Check sheet for the modelled part. Datum: model origin and axes. Units: mm. Face numbers are marked on the shaded views. A direction names the side the tool comes from. Give positions to 0.01 mm unless a question says otherwise; leave off trailing zeros. Order: outer loops, then holes, each group sorted by start corner. A loop starts at its lowest first (then second) coordinate and runs counter-clockwise, first axis right, second up.
from build123d import *

# Parameters (mm, degrees)
F0_R     = 11
F1_DEPTH = 7


with BuildPart() as f1:
    # F0 (on Top) → F1 (new body)
    with BuildSketch(Plane.XY):
        with BuildLine():
            ThreePointArc((-2.577571, 23.56544), (0.124952, 23.151761), (2.813649, 23.647409))
            ThreePointArc((2.813649, 23.647409), (6.73351, 26.656757), (8.219155, 31.369967))
            ThreePointArc((8.219155, 31.369967), (-4.815031, 38.031046), (-2.577571, 23.56544))
        make_face()
        Polygon((6.520027, 31.369967), (3.260014, 25.723457), (-3.260014, 25.723457), (-6.520027, 31.369967), (-3.260014, 37.016476), (3.260014, 37.016476), align=None, mode=Mode.SUBTRACT)
        with BuildLine():
            ThreePointArc((-2.577571, 13.760673), (0.12029, 13.999483), (2.813649, 13.714349))
            Line((2.813649, 13.714349), (2.813649, 23.647409))
            ThreePointArc((2.813649, 23.647409), (0.124952, 23.151761), (-2.577571, 23.56544))
            Line((-2.577571, 23.56544), (-2.577571, 13.760673))
        make_face()
        with BuildLine():
            ThreePointArc((13.205878, -4.648095), (13.800042, -2.357722), (14, 0))
            ThreePointArc((14, 0), (10.848758, 8.848981), (2.813649, 13.714349))
            ThreePointArc((2.813649, 13.714349), (0.12029, 13.999483), (-2.577571, 13.760673))
            ThreePointArc((-2.577571, 13.760673), (-12.063763, 7.103916), (-13.283799, -4.420483))
            ThreePointArc((-13.283799, -4.420483), (-12.184053, -6.895568), (-10.628307, -9.112579))
            ThreePointArc((-10.628307, -9.112579), (-0.12029, -13.999483), (10.470151, -9.293866))
            ThreePointArc((10.470151, -9.293866), (12.063763, -7.103916), (13.205878, -4.648095))
        make_face()
        Circle(F0_R, mode=Mode.SUBTRACT)
        with BuildLine():
            ThreePointArc((-10.628307, -9.112579), (-12.184053, -6.895568), (-13.283799, -4.420483))
            Line((-13.283799, -4.420483), (-21.886082, -9.387013))
            ThreePointArc((-21.886082, -9.387013), (-20.112489, -11.467669), (-19.119484, -14.014962))
            Line((-19.119484, -14.014962), (-10.628307, -9.112579))
        make_face()
        with BuildLine():
            ThreePointArc((-19.119484, -14.014962), (-20.112489, -11.467669), (-21.886082, -9.387013))
            ThreePointArc((-21.886082, -9.387013), (-34.615703, -19.159769), (-18.948033, -15.684983))
            ThreePointArc((-18.948033, -15.684983), (-18.991008, -14.845584), (-19.119484, -14.014962))
        make_face()
        Polygon((-30.427202, -10.038474), (-23.907174, -10.038474), (-20.647161, -15.684983), (-23.907174, -21.331493), (-30.427202, -21.331493), (-33.687215, -15.684983), align=None, mode=Mode.SUBTRACT)
        with BuildLine():
            Line((21.697055, -9.550478), (13.205878, -4.648095))
            ThreePointArc((13.205878, -4.648095), (12.063763, -7.103916), (10.470151, -9.293866))
            Line((10.470151, -9.293866), (19.072433, -14.260396))
            ThreePointArc((19.072433, -14.260396), (19.987538, -11.684092), (21.697055, -9.550478))
        make_face()
        with BuildLine():
            ThreePointArc((35.386343, -15.684983), (30.528337, -8.184504), (21.697055, -9.550478))
            ThreePointArc((21.697055, -9.550478), (19.987538, -11.684092), (19.072433, -14.260396))
            ThreePointArc((19.072433, -14.260396), (26.452184, -23.872979), (35.386343, -15.684983))
        make_face()
        Polygon((23.907174, -21.331493), (20.647161, -15.684983), (23.907174, -10.038474), (30.427202, -10.038474), (33.687215, -15.684983), (30.427202, -21.331493), align=None, mode=Mode.SUBTRACT)
    extrude(amount=F1_DEPTH)


solid = f1.part
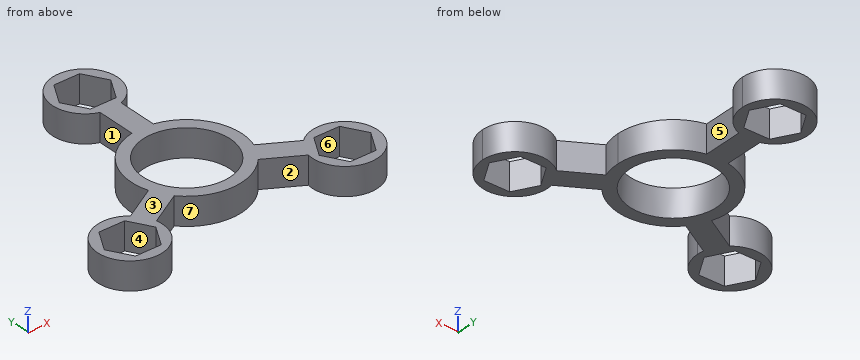
1) Section check C-C, the plane z = 4.5. State how many separate pieces and enclosed holes the cut face has, then the cut area to 3 significant figures.
Recorded:
separate pieces: 1
enclosed holes: 4
area: 693 mm2
2) Section check B-B, the plane y = 9. Record the cut outline in (x, z).
Recorded:
outline: (-10.72, 0) - (-6.32, 0) - (-6.32, 7) - (-10.72, 7) - close; (6.32, 0) - (10.72, 0) - (10.72, 7) - (6.32, 7) - close
3) Material ranges on L1, parallel to Y at x = 0, z = 5.25; L2, parallel to Y at x = -4, z = 5; L3, parallel to Y at x = -3, z = 1.75, recorded low to high.
Recorded:
L1: y = -14 to -11, 11 to 25.72, 37.02 to 39.59
L2: y = -13.42 to -10.25, 10.25 to 13.42, 24.19 to 27.01, 35.73 to 38.55
L3: y = -13.67 to -10.58, 10.58 to 13.67, 23.72 to 25.72, 37.02 to 39.02
4) Set-up check for the marked faces 5, 6 and 7: record each of +Z, -Z, +X, -X, +Y, -Y from which the full face is reachable in a straight line by a thin tool's end or side.
Recorded:
face 5: +Z, -Z, +X
face 6: +Z, -Z
face 7: +Z, -Z, -Y
5) Section check A-A, the plane x = 0. Record the cut outline in (y, z).
Recorded:
outline: (-14, 0) - (-11, 0) - (-11, 7) - (-14, 7) - close; (11, 0) - (25.72, 0) - (25.72, 7) - (11, 7) - close; (37.02, 0) - (39.59, 0) - (39.59, 7) - (37.02, 7) - close
6) Draft check along X on the marked faces 1, 2, 3 and 4. Enter one of: +X half, -X half, draft (parallel to the pull), parting line (faces both ways), or undercut.
Recorded:
face 1: -X half
face 2: undercut
face 3: draft
face 4: undercut
7) Depth check by flat-ended pin: pin 1 Ø1.5 at (y, z) = (-13, 5) entering from +X; pin 2 Ø2 at (x, z) = (26, 4.5) entering from +Y; pin 3 Ø2 at (x, z) = (1.5, 5) entering from -Y. Enter the tip coordinate at first touch or a pass-through.
Recorded:
pin 1: stops at x = 35.16
pin 2: stops at y = -7.47
pin 3: stops at y = -13.99
